```python
from build123d import *

# Parameters (mm, degrees)
BOSS_EXTRUDE1_DEPTH = 2
SKETCH2_R           = 4.25
CUT_EXTRUDE1_DEPTH  = 1
CUT_EXTRUDE4_START  = -8.3
SKETCH8_W           = 3.410115148
SKETCH8_H           = 1.095606144
CUT_EXTRUDE4_DEPTH  = 8.3
BOSS_EXTRUDE4_DEPTH = 0.01
SKETCH9_W           = 0.9
SKETCH9_H           = 3.4
BOSS_EXTRUDE5_DEPTH = 0.3


with BuildPart() as part:
    # Sketch1 → Boss-Extrude1 (new body)
    with BuildSketch(Plane(origin=(0, 0, 0), x_dir=(1, 0, 0), z_dir=(0, 1, 0))):
        Polygon((-4.15, 4.15), (4.15, 4.15), (4.15, -2.402631579), (2.402631579, -4.15), (-2.315263158, -4.15), (-4.15, -2.315263158), align=None)
    extrude(amount=BOSS_EXTRUDE1_DEPTH)

    # Sketch2 → Cut-Extrude1 (cut)
    with BuildSketch(Plane(origin=(0, 2, 0), x_dir=(1, 0, 0), z_dir=(0, 1, 0))):
        Circle(SKETCH2_R)
    extrude(amount=-CUT_EXTRUDE1_DEPTH, mode=Mode.SUBTRACT)

    # Sketch8 → Cut-Extrude4 (cut)
    with BuildSketch(Plane.ZY.offset(4.15).offset(CUT_EXTRUDE4_START)):
        with Locations((2.621572713, 1.765165498)):
            Rectangle(SKETCH8_W, SKETCH8_H)
    extrude(amount=CUT_EXTRUDE4_DEPTH, mode=Mode.SUBTRACT)

    # Sketch5 → Revolve1 (revolve)
    with BuildSketch(Plane.XY, mode=Mode.PRIVATE) as revolve1_sk:
        with BuildLine():
            Line((0, 1), (-4, 1))
            Line((-4, 1), (-4, 2.5))
            ThreePointArc((-4, 2.5), (-3.9, 2.6), (-4, 2.7))
            Line((-4, 2.7), (-4, 10.05))
            ThreePointArc((-4, 10.05), (-3.956066017, 10.156066017), (-3.85, 10.2))
            Line((-3.85, 10.2), (0, 10.2))
            Line((0, 10.2), (0, 1))
        make_face()
    revolve(revolve1_sk.sketch.rotate(Axis((0, 10.2, 0), (0, -1, 0)), 270), axis=Axis((0, 10.2, 0), (0, -1, 0)))

    # Sketch6 → Boss-Extrude4 (add)
    with BuildSketch(Plane(origin=(0, 10.2, 0), x_dir=(1, 0, 0), z_dir=(0, 1, 0))):
        with BuildLine():
            Line((-3.403621507, 1.799405635), (3.403621507, 1.799405635))
            ThreePointArc((3.403621507, 1.799405635), (0, 3.85), (-3.403621507, 1.799405635))
        make_face()
    extrude(amount=BOSS_EXTRUDE4_DEPTH)

    # Sketch9 → Boss-Extrude5 (add)
    with BuildSketch(Plane.XZ):
        with Locations((0, -3.25)):
            Rectangle(SKETCH9_W, SKETCH9_H)
        with Locations((0, 3.25)):
            Rectangle(SKETCH9_W, SKETCH9_H)
    extrude(amount=BOSS_EXTRUDE5_DEPTH)


solid = part.part
```
Work out the finished part from the listing and answer in its coordinate system (mm). A direction names the side the tool comes from. Coordinates: 2 decimals unless noted, no trailing zeros. Loops run counter-clockwise (first coordinate to the right, second up) from the corner with the lowest first, then second, coordinate; pieces in that order, holes last. Notation, with made-up numbers: (-14.75, -19) -> (9.25, -19) arc R32 ccw to (9.25, 19) -> close; hole circle Ø1 at (71.25, 15.25). An arc over 180 degrees is marked (long way). Answer as CSV lines item,"result".
Q1. Find the intervals of material crossed by probe 1 along Y at (x, z) = (-1.5, 2); probe 2 along Y at (x, z) = (2.25, 3.75); probe 3 along X at (y, z) = (9.5, -1), in increasing order.
Findings:
probe 1,"y = 0 to 10.2"
probe 2,"y = 0 to 1.22"
probe 3,"x = -3.87 to 3.87"
Q2. The part is cut by section C-C on y = 3. Write down the section's boundary in (x, z), and give its area (3 significant figures).
Findings:
outline,"circle Ø8 at (0, 0)"
area,"50.3 mm²"
Q3. For a pull along Z with two mould halves and no side action, classify faces 1 (the face through (-2.98, 1.51, -3.03)), 2 (the face through (-3.22, 0.6, 3.245)), 3 (the face through (-0.1, 0.8, -4.15)), 4 (the face through (0, -0.3, -3)) as +Z half, -Z half, draft (parallel to the pull), parting line (faces both ways), or undercut.
Findings:
face 1,"undercut"
face 2,"+Z half"
face 3,"-Z half"
face 4,"draft"
Q4. The part is cut by section B-B on z = 0. Write down the section's boundary in (x, y), and give its area (3 significant figures).
Findings:
outline,"(-4.15, 0) -> (4.15, 0) -> (4.15, 1) -> (4, 1) -> (4, 2.5) arc R0.1 cw to (4, 2.7) -> (4, 10.05) arc R0.15 ccw to (3.85, 10.2) -> (-3.85, 10.2) arc R0.15 ccw to (-4, 10.05) -> (-4, 2.7) arc R0.1 cw to (-4, 2.5) -> (-4, 1) -> (-4.15, 1) -> close"
area,"81.9 mm²"
Q5. A tool of negligible diameter and unlimited length cuts with its end or side. For faces 5 (the face through (0.1, 0.6, 4.15)), 6 (the face through (-3.12, 1.217, 3.12)), 7 (the face through (3.03, 1.51, -2.98)), 8 (the face through (-3.2, 2, -3.3)), from which of +Z, -Z, +X, -X, +Y, -Y can it reach the whole face along a straight path? Write none if from no direction.
Findings:
face 5,"+Z, +X, -X, +Y"
face 6,"+Z, -X, +Y"
face 7,"+Y"
face 8,"-Z, -X, +Y"
Q6. Each of these flat-tipped pins is pushed along its axis until it touches: pin 1 (3 mm diameter, centred on x = 0, z = 1.5, fed in from +Y); pin 2 (1.6 mm diameter, centred on x = 0.5, y = 1.5, fed in from -Z); pin 3 (1.5 mm diameter, centred on y = 8, z = -1, fed in from -X); pin 4 (1.3 mm diameter, centred on x = 0, y = 0.5, fed in from +Z). Where does it stop, or does it pass through?
Findings:
pin 1,"stops at y = 10.2"
pin 2,"stops at z = -4.15"
pin 3,"stops at x = -3.99"
pin 4,"stops at z = 4.95"
